Job drawing, mm, ordinate dimensions from the low corner. One solid piece. A direction names the side the tool comes from. Give positions to 0.01 mm unless a question says otherwise; leave off trailing zeros. Loops run counter-clockwise (first coordinate to the right, second up) from the corner with the lowest first, then second, coordinate; pieces in that order, holes last. Notation, with made-up numbers: (-22.75, 6.5) -> (-4.75, 6.5) arc R25 cw to (-4.75, 45.5) -> close; hole circle Ø10 at (85.5, 75.5). An arc over 180 degrees is marked (long way). Answer as a JSON object with one key per item and string values. Group by question number.
Q1. Band-saw the part on A-A, the plane x = 74. Write the cut outline in (y, z), plus the area to 3 significant figures.
Q2. Band-saw the part on D-D, the plane y = 40.5. Write the cut outline in (x, z).
Q3. Two-plate mould, pull along Z, no slides. Class the marked faces 1, 2, 3 and 4: pulls with the +Z half, pulls with the -Z half, needs draft (parallel to the pull), parting line crosses it, or undercut.
Q4. Wall check: probe 1 along Y at (x, z) = (38.5, 16); probe 2 along Y at (x, z) = (28.5, 50). Give the ranges that are in metal, low to high. Write a range as from..to.
Q5. Band-saw the part on C-C, the plane x = 28. Write the cut outline in (y, z).
Q6. Drop flat-ended pins along their axis: pin 1 (3 mm diameter, centred on x = 19.5, z = 13, fed in from +Y); pin 2 (2 mm diameter, centred on x = 12, y = 39, fed in from +Z); pin 3 (14.5 mm diameter, centred on y = 49.5, z = 17, fed in from +X). Give the stop position or say it passes through.
Q7. Band-saw the part on B-B, the plane z = 10. Write the cut outline in (x, y).
Q8. Tool access for the marked faces 5, 6 and 7: list every direction of +Z, -Z, +X, -X, +Y, -Y with a clear straight run to the whole face (end or side of a thin tool).
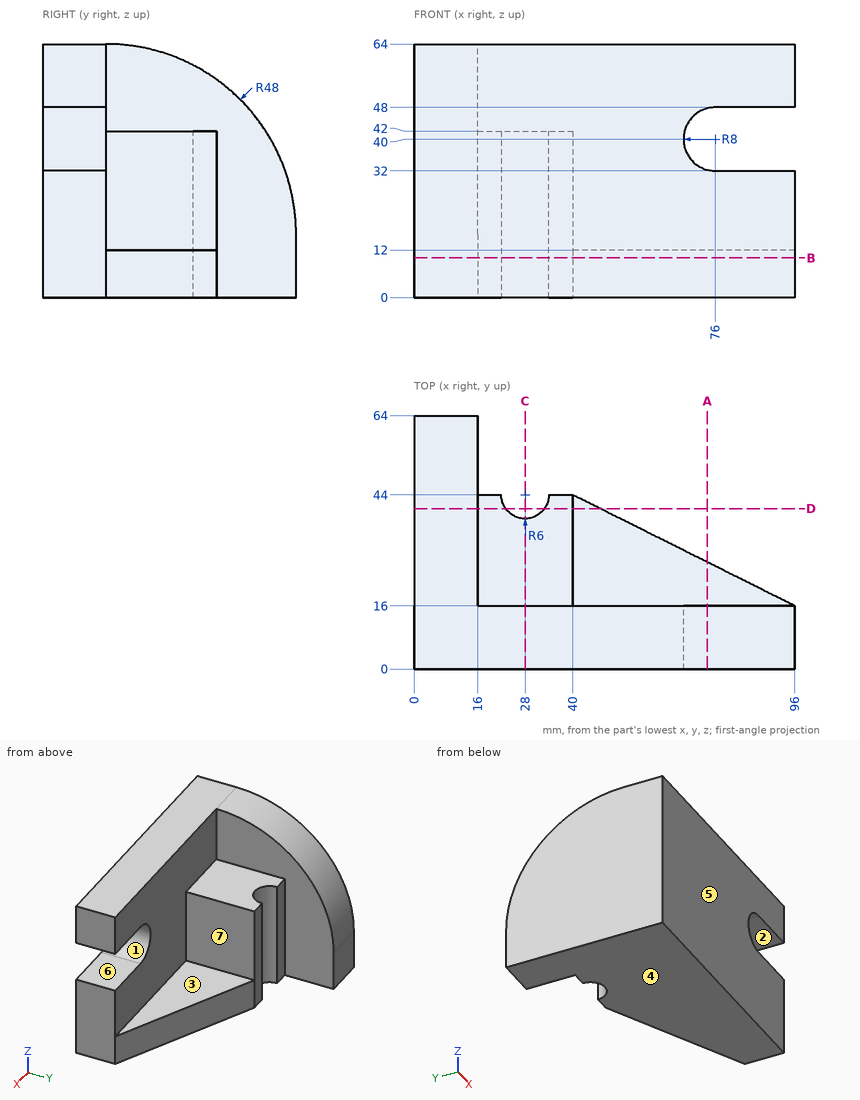
Worked answers:
{
 "1": {"outline": "(0, 0) -> (27, 0) -> (27, 12) -> (16, 12) -> (16, 32.25) -> (0, 32.25) -> close; (0, 47.75) -> (16, 47.75) -> (16, 64) -> (0, 64) -> close", "area": "908 mm2"},
 "2": {"outline": "(0, 0) -> (23.13, 0) -> (23.13, 42) -> (16, 42) -> (16, 57.28) -> (0, 57.28) -> close; (32.87, 0) -> (47, 0) -> (47, 12) -> (40, 12) -> (40, 42) -> (32.87, 42) -> close"},
 "3": {"face 1": "undercut", "face 2": "undercut", "face 3": "pulls with the +Z half", "face 4": "pulls with the -Z half"},
 "4": {"probe 1": "0..44", "probe 2": "0..16"},
 "5": {"outline": "(0, 0) -> (38, 0) -> (38, 42) -> (16, 42) -> (16, 64) -> (0, 64) -> close"},
 "6": {"pin 1": "y = 44", "pin 2": "z = 58.66", "pin 3": "x = 40"},
 "7": {"outline": "(0, 0) -> (96, 0) -> (96, 16) -> (40, 44) -> (34, 44) arc R6 cw to (22, 44) -> (16, 44) -> (16, 64) -> (0, 64) -> close"},
 "8": {"face 5": "+Z, -Z, +X, -X, -Y", "face 6": "+X, +Y, -Y", "face 7": "+Z, +X, +Y"}
}
